from build123d import *

# Parameters (mm, degrees)
BOSS_EXTRUDE1_DEPTH = 6
SKETCH3_R           = 1.4
CUT_EXTRUDE1_DEPTH  = 20
SKETCH4_R           = 1.5
CUT_EXTRUDE2_DEPTH  = 200


with BuildPart() as part:
    # Sketch1 → Boss-Extrude1 (new body)
    with BuildSketch(Plane(origin=(0, 0, 0), x_dir=(1, 0, 0), z_dir=(0, 1, 0))):
        with BuildLine():
            Line((5.807869676, 47.103606084), (12.202893506, 47.103606084))
            ThreePointArc((12.202893506, 47.103606084), (12.865186965, 46.85285062), (13.195333016, 46.226340832))
            Line((13.195333016, 46.226340832), (20.148830597, -10))
            Line((20.148830597, -10), (-1.041666667, -10))
            Line((-1.041666667, -10), (4.813251268, 46.207212169))
            ThreePointArc((4.813251268, 46.207212169), (5.13839454, 46.846440549), (5.807869676, 47.103606084))
        make_face()
        with BuildLine():
            Line((9.674718252, 42.103606084), (15.291737007, -3.315897879))
            ThreePointArc((15.291737007, -3.315897879), (14.926944544, -4.493440189), (13.803077741, -5))
            Line((13.803077741, -5), (5.165175568, -5))
            ThreePointArc((5.165175568, -5), (4.050923871, -4.504212704), (3.673247955, -3.344590874))
            Line((3.673247955, -3.344590874), (8.407435138, 42.103606084))
            Line((8.407435138, 42.103606084), (9.674718252, 42.103606084))
        make_face(mode=Mode.SUBTRACT)
    extrude(amount=BOSS_EXTRUDE1_DEPTH)

    # Sketch3 → Cut-Extrude1 (cut)
    with BuildSketch(Plane(origin=(0, 0, -47.103606084), x_dir=(-1, 0, 0), z_dir=(0, 0, -1))):
        with Locations((-9.005381591, 3)):
            Circle(SKETCH3_R)
    extrude(amount=-CUT_EXTRUDE1_DEPTH, mode=Mode.SUBTRACT)

    # Sketch4 → Cut-Extrude2 (cut)
    with BuildSketch(Plane.XY):
        with Locations(Location((9.445211312, 3, 0), (0, 0, 180))):
            Circle(SKETCH4_R)
    extrude(amount=CUT_EXTRUDE2_DEPTH, mode=Mode.SUBTRACT)


solid = part.part
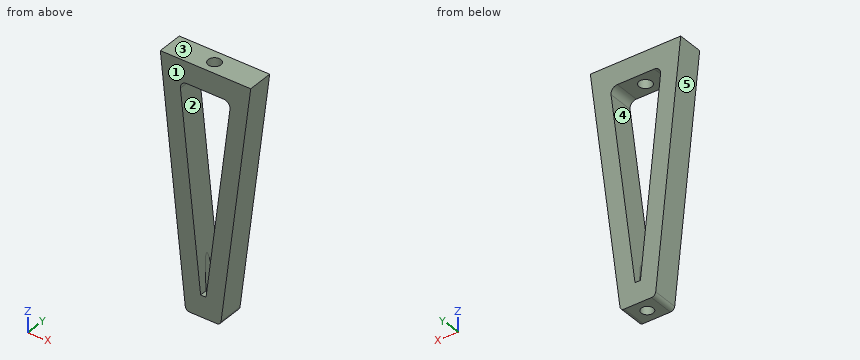
Geometry check sheet. Reference: the model listing, model coordinates, mm. Face numbers are marked on the shaded views. A direction names the side the tool comes from. Round coordinates to 2 decimals unless told otherwise and drop trailing zeros. Order: outer loops, then holes, each group sorted by start corner. A loop starts at its lowest first (then second) coordinate and runs counter-clockwise, first axis right, second up. Notation, with made-up numbers: M -11.75,60 L 9.25,60 A21 cw 9.25,88 Z; hole C 15,89.5 d11. An arc over 180 degrees is marked long. Answer in a Markdown table with one row per item. Add a question column.
Item 1: Draft check along Z on the marked faces 3, 4 and 5. Enter one of: released by +Z, released by -Z, zero draft, split by the parting line, or undercut.
Item 2: Sectioned sample at B-B, the plane y = 0.5. Enter the section's corners in (x, z).
Item 3: Sectioned sample at A-A, the plane y = 3. Enter the section's corners in (x, z), plus the area to 3 significant figures.
Item 4: Material ranges on L1, parallel to X at y = 0.5, z = -37.5; L2, parallel to Y at x = 10.5, z = 6.5; L3, parallel to X at y = 3, z = -43.75, recorded low to high. Write a range as [from, to].
Item 5: Sectioned sample at C-C, the plane z = -3. Enter the section's corners in (x, y).
Item 6: Set-up check for the marked faces 1 and 2: record each of +Z, -Z, +X, -X, +Y, -Y from which the full face is reachable in a straight line by a thin tool's end or side.
Item 7: Sectioned sample at D-D, the plane x = 0.5. Enter the section's corners in (y, z).
Filled in:
| question | item | result |
|---|---|---|
| 1 | face 3 | released by +Z |
| 1 | face 4 | undercut |
| 1 | face 5 | released by -Z |
| 2 | outline | M -1.04,10 L 4.81,-46.21 A1 ccw 5.81,-47.1 L 12.2,-47.1 A1 ccw 13.2,-46.23 L 20.15,10 Z; hole M 3.67,3.34 L 8.41,-42.1 L 9.67,-42.1 L 15.29,3.32 A1.5 ccw 13.8,5 L 5.17,5 A1.5 ccw Z |
| 3 | outline | M -1.04,10 L 4.81,-46.21 A1 ccw 5.81,-47.1 L 7.61,-47.1 L 7.61,-34.4 L 3.67,3.34 A1.5 cw 5.17,5 L 7.95,5 L 7.95,10 Z; M 10.41,-47.1 L 12.2,-47.1 A1 ccw 13.2,-46.23 L 20.15,10 L 10.95,10 L 10.95,5 L 13.8,5 A1.5 cw 15.29,3.32 L 10.41,-36.2 Z |
| 3 | area | 493 mm² |
| 4 | L1 | x = [3.91, 7.93], [10.24, 14.27] |
| 4 | L2 | y = [0, 1.93], [4.07, 6] |
| 4 | L3 | x = [4.56, 7.61], [10.41, 13.5] |
| 5 | outline | M 0.31,0 L 4.33,0 L 4.33,6 L 0.31,6 Z; M 14.51,0 L 18.54,0 L 18.54,6 L 14.51,6 Z |
| 6 | face 1 | +Z, -Z, +X, -X, -Y |
| 6 | face 2 | +Y, -Y |
| 7 | outline | M 0,-4.8 L 6,-4.8 L 6,10 L 0,10 Z |
